from build123d import *

# Parameters (mm, degrees)
SKETCH1_R           = 1.6
BOSS_EXTRUDE1_DEPTH = 4
CUT_EXTRUDE1_DEPTH  = 2
CUT_EXTRUDE2_DEPTH  = 1.5
SKETCH5_R           = 4
BOSS_EXTRUDE2_DEPTH = 1.5
SKETCH8_R           = 1.5
CUT_EXTRUDE3_DEPTH  = 52.119956964
CIRPATTERN1_COUNT   = 4
FILLET1_R           = 3
FILLET1_R_2         = 2
FILLET2_R           = 30


with BuildPart() as part:
    # Sketch1 → Boss-Extrude1 (new body)
    with BuildSketch(Plane(origin=(0, 0, 0), x_dir=(1, 0, 0), z_dir=(0, 1, 0))):
        Polygon((12.5, 35), (-12.5, 35), (-23.334523779, 36.062445841), (-36.062445841, 23.334523779), (-35, 12.5), (-35, -12.5), (-36.062445841, -23.334523779), (-23.334523779, -36.062445841), (-12.5, -35), (12.5, -35), (23.334523779, -36.062445841), (36.062445841, -23.334523779), (35, -12.5), (35, 12.5), (36.062445841, 23.334523779), (23.334523779, 36.062445841), align=None)
        with Locations(Location((22.627416998, 31.112698372, 0), (0, 0, 270))):
            Circle(SKETCH1_R, mode=Mode.SUBTRACT)
        with Locations(Location((31.112698372, 22.627416998, 0), (0, 0, 270))):
            Circle(SKETCH1_R, mode=Mode.SUBTRACT)
        with Locations(Location((22.627416998, -31.112698372, 0), (0, 0, 270))):
            Circle(SKETCH1_R, mode=Mode.SUBTRACT)
        with Locations(Location((31.112698372, -22.627416998, 0), (0, 0, 270))):
            Circle(SKETCH1_R, mode=Mode.SUBTRACT)
        with Locations(Location((-31.112698372, -22.627416998, 0), (0, 0, 270))):
            Circle(SKETCH1_R, mode=Mode.SUBTRACT)
        with Locations(Location((-22.627416998, -31.112698372, 0), (0, 0, 270))):
            Circle(SKETCH1_R, mode=Mode.SUBTRACT)
        with Locations(Location((-22.627416998, 31.112698372, 0), (0, 0, 270))):
            Circle(SKETCH1_R, mode=Mode.SUBTRACT)
        with Locations(Location((-31.112698372, 22.627416998, 0), (0, 0, 270))):
            Circle(SKETCH1_R, mode=Mode.SUBTRACT)
    extrude(amount=BOSS_EXTRUDE1_DEPTH)

    # Sketch2 → Cut-Extrude1 (cut)
    with BuildSketch(Plane(origin=(0, 4, 0), x_dir=(1, 0, 0), z_dir=(0, 1, 0))):
        Polygon((-17.669047558, 29), (17.669047558, 29), (29, 17.669047558), (29, -17.669047558), (17.669047558, -29), (-17.669047558, -29), (-29, -17.669047558), (-29, 17.669047558), align=None)
    extrude(amount=-CUT_EXTRUDE1_DEPTH, mode=Mode.SUBTRACT)

    # Sketch4 → Cut-Extrude2 (cut)
    with BuildSketch(Plane(origin=(0, 2, 0), x_dir=(1, 0, 0), z_dir=(0, 1, 0))):
        with BuildLine():
            Line((-24.079215521, 13.567556979), (-16.079215521, 6.899529803))
            ThreePointArc((-16.079215521, 6.899529803), (-15.283167889, 5.867388581), (-15, 4.595058717))
            Line((-15, 4.595058717), (-15, -4.595058717))
            ThreePointArc((-15, -4.595058717), (-15.283167889, -5.867388581), (-16.079215521, -6.899529803))
            Line((-16.079215521, -6.899529803), (-24.079215521, -13.567556979))
            ThreePointArc((-24.079215521, -13.567556979), (-27.272329864, -13.979918004), (-29, -11.263085893))
            Line((-29, -11.263085893), (-29, 11.263085893))
            ThreePointArc((-29, 11.263085893), (-27.272329864, 13.979918004), (-24.079215521, 13.567556979))
        make_face()
        with BuildLine():
            Line((-11.263085893, 29), (11.263085893, 29))
            ThreePointArc((11.263085893, 29), (13.979918004, 27.272329864), (13.567556979, 24.079215521))
            Line((13.567556979, 24.079215521), (6.899529803, 16.079215521))
            ThreePointArc((6.899529803, 16.079215521), (5.867388581, 15.283167889), (4.595058717, 15))
            Line((4.595058717, 15), (-4.595058717, 15))
            ThreePointArc((-4.595058717, 15), (-5.867388581, 15.283167889), (-6.899529803, 16.079215521))
            Line((-6.899529803, 16.079215521), (-13.567556979, 24.079215521))
            ThreePointArc((-13.567556979, 24.079215521), (-13.979918004, 27.272329864), (-11.263085893, 29))
        make_face()
        with BuildLine():
            Line((29, 11.263085893), (29, -11.263085893))
            ThreePointArc((29, -11.263085893), (27.272329864, -13.979918004), (24.079215521, -13.567556979))
            Line((24.079215521, -13.567556979), (16.079215521, -6.899529803))
            ThreePointArc((16.079215521, -6.899529803), (15.283167889, -5.867388581), (15, -4.595058717))
            Line((15, -4.595058717), (15, 4.595058717))
            ThreePointArc((15, 4.595058717), (15.283167889, 5.867388581), (16.079215521, 6.899529803))
            Line((16.079215521, 6.899529803), (24.079215521, 13.567556979))
            ThreePointArc((24.079215521, 13.567556979), (27.272329864, 13.979918004), (29, 11.263085893))
        make_face()
        with BuildLine():
            Line((11.263085893, -29), (-11.263085893, -29))
            ThreePointArc((-11.263085893, -29), (-13.979918004, -27.272329864), (-13.567556979, -24.079215521))
            Line((-13.567556979, -24.079215521), (-6.899529803, -16.079215521))
            ThreePointArc((-6.899529803, -16.079215521), (-5.867388581, -15.283167889), (-4.595058717, -15))
            Line((-4.595058717, -15), (4.595058717, -15))
            ThreePointArc((4.595058717, -15), (5.867388581, -15.283167889), (6.899529803, -16.079215521))
            Line((6.899529803, -16.079215521), (13.567556979, -24.079215521))
            ThreePointArc((13.567556979, -24.079215521), (13.979918004, -27.272329864), (11.263085893, -29))
        make_face()
    extrude(amount=-CUT_EXTRUDE2_DEPTH, mode=Mode.SUBTRACT)

    # Sketch5 → Boss-Extrude2 (add)
    with BuildSketch(Plane(origin=(0, 2, 0), x_dir=(1, 0, 0), z_dir=(0, 1, 0))):
        with Locations(Location((15.25, 15.25, 0), (0, 0, 90))):
            Circle(SKETCH5_R)
    boss_extrude2 = extrude(amount=BOSS_EXTRUDE2_DEPTH)

    # Sketch8 → Cut-Extrude3 (cut, through all)
    with BuildSketch(Plane(origin=(0, 3.5, 0), x_dir=(1, 0, 0), z_dir=(0, 1, 0))):
        with Locations(Location((15.25, 15.25, 0), (0, 0, 270))):
            Circle(SKETCH8_R)
    cut_extrude3 = extrude(amount=-CUT_EXTRUDE3_DEPTH, mode=Mode.SUBTRACT)

    # CirPattern1: Boss-Extrude2, Cut-Extrude3 ×4 about axis
    cirpattern1_axis = Axis((0, 0, 0), (0, 1, 0))
    add([boss_extrude2.rotate(cirpattern1_axis, i * 360 / CIRPATTERN1_COUNT) for i in range(1, CIRPATTERN1_COUNT)])
    add([cut_extrude3.rotate(cirpattern1_axis, i * 360 / CIRPATTERN1_COUNT) for i in range(1, CIRPATTERN1_COUNT)], mode=Mode.SUBTRACT)

    # Fillet1
    # the kernel refuses this fillet: 3, 2 mm, written as the material it adds along each edge
    with BuildSketch(Plane(origin=(-15.25, 2, -15.25), x_dir=(-1, 0, 0), z_dir=(0, 0, -1))) as fillet1_piece_1:
        with BuildLine():
            CenterArc((6.598076211, 3), FILLET1_R, 210, 60)
            Line((4, 1.5), (3.948038476, 1.47))
            ThreePointArc((3.948038476, 1.47), (3.94, 0.75), (3.94, 0))
            Line((3.94, 0), (4, -0.06))
            Line((4, -0.06), (6.598076211, -0.06))
            Line((6.598076211, -0.06), (6.598076211, 0))
        make_face()
    revolve(axis=Axis((-15.25, 2, -15.25), (0, 1, 0)))
    with BuildSketch(Plane(origin=(-15.25, 2, 15.25), x_dir=(0, 0, 1), z_dir=(-1, 0, 0))) as fillet1_piece_2:
        with BuildLine():
            CenterArc((6.598076211, 3), FILLET1_R, 210, 60)
            Line((4, 1.5), (3.948038476, 1.47))
            ThreePointArc((3.948038476, 1.47), (3.94, 0.75), (3.94, 0))
            Line((3.94, 0), (4, -0.06))
            Line((4, -0.06), (6.598076211, -0.06))
            Line((6.598076211, -0.06), (6.598076211, 0))
        make_face()
    revolve(axis=Axis((-15.25, 2, 15.25), (0, 1, 0)))
    with BuildSketch(Plane(origin=(15.25, 2, 15.25), x_dir=(1, 0, 0), z_dir=(0, 0, 1))) as fillet1_piece_3:
        with BuildLine():
            CenterArc((6.598076211, 3), FILLET1_R, 210, 60)
            Line((4, 1.5), (3.948038476, 1.47))
            ThreePointArc((3.948038476, 1.47), (3.94, 0.75), (3.94, 0))
            Line((3.94, 0), (4, -0.06))
            Line((4, -0.06), (6.598076211, -0.06))
            Line((6.598076211, -0.06), (6.598076211, 0))
        make_face()
    revolve(axis=Axis((15.25, 2, 15.25), (0, 1, 0)))
    with BuildSketch(Plane(origin=(15.25, 2, -15.25), x_dir=(0, 0, -1), z_dir=(1, 0, 0))) as fillet1_piece_4:
        with BuildLine():
            CenterArc((5.936491673, 2), FILLET1_R_2, 194.477512186, 75.522487814)
            Line((4, 1.5), (3.961270167, 1.49))
            ThreePointArc((3.961270167, 1.49), (3.96, 0.75), (3.96, 0))
            Line((3.96, 0), (4, -0.04))
            Line((4, -0.04), (5.936491673, -0.04))
            Line((5.936491673, -0.04), (5.936491673, 0))
        make_face()
    revolve(axis=Axis((15.25, 2, -15.25), (0, 1, 0)))

    # Fillet2
    # the kernel refuses this fillet: 30 mm, written as the material it adds along each edge
    with BuildSketch(Plane(origin=(-12.5, 0, -35), x_dir=(1, 0, 0), z_dir=(0, 1, 0)), Plane(origin=(-12.5, 0, 35), x_dir=(-0.9952264052892464, 0, 0.09759304388656438), z_dir=(0, 1, 0)), Plane(origin=(-35, 0, 12.5), x_dir=(0, 0, -1), z_dir=(0, 1, 0)), Plane(origin=(-35, 0, -12.5), x_dir=(-0.09759304388656037, 0, -0.9952264052892466), z_dir=(0, 1, 0))) as fillet2_piece_1:
        with BuildLine():
            CenterArc((FILLET2_R * 0.0489132680017, FILLET2_R), FILLET2_R, 264.399415997, 5.600584003)
            Line((-FILLET2_R * 0.0486797758843, FILLET2_R * 0.0047735947107), (0, 0))
            Line((0, 0), (FILLET2_R * 0.0489132680017, 0))
        make_face()
    extrude(amount=4)
    with BuildSketch(Plane(origin=(12.5, 0, -35), x_dir=(-1, 0, 0), z_dir=(0, 1, 0)), Plane(origin=(35, 0, -12.5), x_dir=(0.09759304388597856, 0, -0.9952264052893037), z_dir=(0, 1, 0)), Plane(origin=(35, 0, 12.5), x_dir=(0, 0, -1), z_dir=(0, 1, 0)), Plane(origin=(12.5, 0, 35), x_dir=(0.9952264052893038, 0, 0.09759304388597881), z_dir=(0, 1, 0))) as fillet2_piece_2:
        with BuildLine():
            CenterArc((FILLET2_R * 0.048913268002, -FILLET2_R), FILLET2_R, 90, 5.600584003)
            Line((-FILLET2_R * 0.0486797758846, -FILLET2_R * 0.00477359471075), (0, 0))
            Line((0, 0), (FILLET2_R * 0.048913268002, 0))
        make_face()
    extrude(amount=4)


solid = part.part
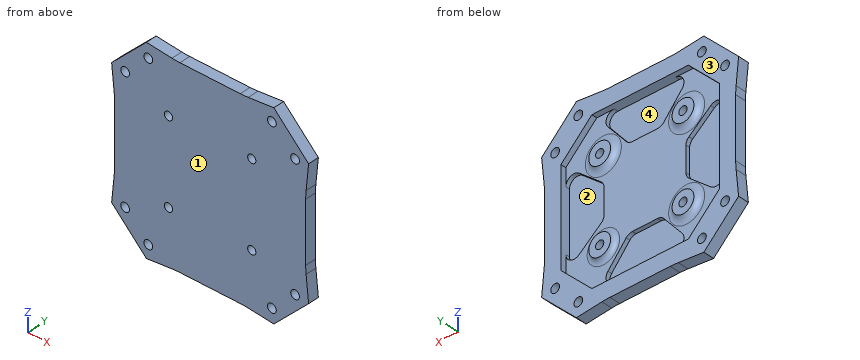
Can you work these out from the model? Positions are in its coordinate system, mm. Face numbers are marked on the shaded views. A direction names the side the tool comes from. Round coordinates to 2 decimals unless told otherwise and drop trailing zeros. Write each loop counter-clockwise with the first axis right and the second up, starting at its lowest first coordinate (ties: lowest second). Pieces come first, ordered by that corner, then holes. Notation, with made-up numbers: M -35.75,82 L -15.75,82 A18 ccw -15.75,109 Z; hole C -14.5,71.5 d9. An arc over 180 degrees is marked long. Use CSV: the item, a comma, the result in double quotes.
(1) Imagine slicing it at A-A (x = -1). Write out the boundary of the cut face in (y, z), plus the area to 3 significant figures.
Check values:
outline,"M 0,-35 L 4,-35 L 4,-29 L 0.5,-29 L 0.5,-15 L 2,-15 L 2,15 L 0.5,15 L 0.5,29 L 4,29 L 4,35 L 0,35 Z"
area,"122 mm^2"
(2) Imagine slicing it at C-C (x = -27). Write out the boundary of the cut face in (y, z), plus the area to 3 significant figures.
Check values:
outline,"M 0,-32.4 L 4,-32.4 L 4,-19.67 L 2,-19.67 L 2,-14.09 L 0.5,-14.09 L 0.5,14.09 L 2,14.09 L 2,19.67 L 4,19.67 L 4,32.4 L 0,32.4 Z"
area,"138 mm^2"
(3) Imagine slicing it at B-B (y = 1.2). Count the separate pieces of the cut face and the enclosed holes in it, plus the area to 3 significant figures.
Check values:
separate pieces,"1"
enclosed holes,"16"
area,"3,380 mm^2"
(4) We'd pull the mould along X, two halves only. Please class the marked faces 1 and 2: +X half, -X half, draft (parallel to the pull), parting line (faces both ways), or undercut.
Check values:
face 1,"draft"
face 2,"undercut"
(5) On a 3-axis mill with a long thin cutter (end or side, diameter ignored), from which of +Z, -Z, +X, -X, +Y, -Y can I reach the whole of each face in a straight line? I mean the marked faces 3 and 4. Say none if no direction works.
Check values:
face 3,"+Z, -Z, +X, -X, +Y"
face 4,"+Y"
(6) I need wall thicknesses on line 1 along X through (y, z) = (1.8, 3); line 2 along Z through (x, y) = (3.5, 2.9). Which ranges of each line are inside material? Lowest first, please.
Check values:
line 1,"-35 to -29, -15 to 15, 29 to 35"
line 2,"-35 to -29, 29 to 35"
(7) I'm going to push flat-ended pins straight in: pin 1 (2 mm diameter, centred on y = 1, z = 1.5, fed in from +X); pin 2 (12 mm diameter, centred on x = -2, z = 18.5, fed in from -Y); pin 3 (2.5 mm diameter, centred on x = -14, z = -15.5, fed in from +Y); pin 4 (1.6 mm diameter, centred on x = -1, y = 1.5, fed in from -Z). Where does each tip first touch, or does it pass through?
Check values:
pin 1,"x = 35"
pin 2,"y = 0"
pin 3,"y = 3.5"
pin 4,"z = -35"
